Could you check a few things on this model? Use its own coordinates, in mm. Give positions to 0.01 mm unless a question says otherwise; leave off trailing zeros. Loops run counter-clockwise (first coordinate to the right, second up) from the corner with the lowest first, then second, coordinate; pieces in that order, holes last. Notation, with made-up numbers: M 33,13.25 L 49,13.25 A19 cw 49,18.25 Z; hole C -28,58.25 d4. An arc over 180 degrees is marked long. Use a Markdown table: item, result. Add a question column.
1) Suppose I cut it at D-D on y = -2. List the corners of the cut face in (x, z) for me, and give its area (3 significant figures).
2) If I drill on line 1 along Y through (x, z) = (6, 0); line 2 along Z through (x, y) = (3, 0), over which ranges is the centre line in solid material (lowest first)? Write a range as [from, to].
3) Suppose I cut it at C-C on x = 14. List the corners of the cut face in (y, z) for me.
4) Will these pins go through, and if not, where does the flat tip stop? pin 1 Ø2 at (x, y) = (13, -0.5) entering from +Z; pin 2 Ø2 at (x, y) = (4.5, -3) entering from +Z; pin 3 Ø2 at (x, z) = (10.5, 0.5) entering from +Y; pin 4 Ø0.6 at (x, z) = (10, 0) entering from -Y.
5) Suppose I cut it at B-B on z = 1.75. List the corners of the cut face in (x, y) for me, and give its area (3 significant figures).
6) Suppose I cut it at A-A on y = 0. List the corners of the cut face in (x, z) for me.
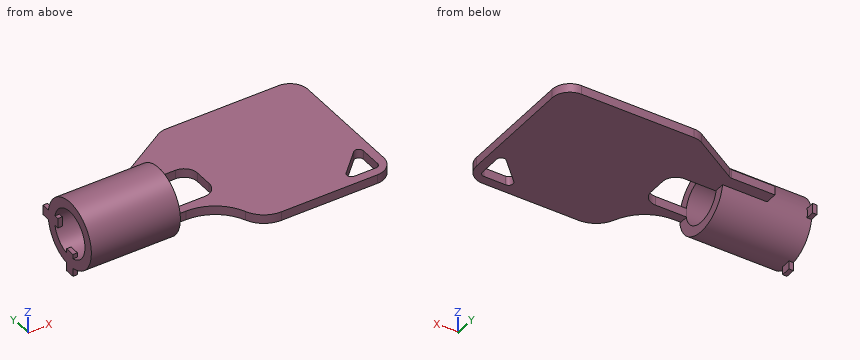
Autodesk Inventor part; units mm, degrees
ref_plane "k_to_1_XY" through (0, 0, 0) normal (1, 0, 0) x (0, 0, -1)
ref_plane "k_to_1_YZ" through (0, 0, 0) normal (0, 0, -1) x (0, 1, 0)
ref_plane "k_to_1_ZX" through (0, 0, 0) normal (0, 1, 0) x (1, 0, 0)
sketch "Sketch_1" plane through (0, 0, 0) normal (1, 0, 0) x (0, 1, 0)
  circle A0 centre (0, 0) radius 3.707
  circle A1 centre (0, 0) radius 2.607
extrude "Extrusion1" add sketch "Sketch_1" along normal blind 10
sketch "Sketch_2" plane through (0, 0, 0) normal (1, 0, 0) x (0, 1, 0)
  line L0 (2.0509, 0.55) -> (2.0509, -0.55)
  line L1 (2.0509, -0.55) -> (4.6009, -0.55)
  line L2 (4.6009, -0.55) -> (4.6009, 0.55)
  line L3 (4.6009, 0.55) -> (2.0509, 0.55)
extrude "Extrusion2" add sketch "Sketch_2" along normal blind 0.5
sketch "Sketch_3" plane through (0, 0, 0) normal (1, 0, 0) x (0, 1, 0)
  line L0 (0.55, -2.0509) -> (-0.55, -2.0509)
  line L1 (-0.55, -2.0509) -> (-0.55, -4.6009)
  line L2 (-0.55, -4.6009) -> (0.55, -4.6009)
  line L3 (0.55, -4.6009) -> (0.55, -2.0509)
extrude "Extrusion3" add sketch "Sketch_3" along normal blind 0.5
sketch "Sketch_4" plane through (0, 0, 0) normal (0, 0, 1) x (1, 0, 0)
  line L0 (5, 5) -> (5, 3.5)
  line L1 (5, 3.5) -> (10, 3.5)
  line L2 (10, 3.5) -> (10, 2.5)
  line L3 (10, 2.5) -> (13.5, 2.5)
  arc A0 (15, 1) -> (13.5, 2.5) centre (13.5, 1) ccw
  line L4 (15, 1) -> (15, -1)
  arc A1 (13.5, -2.5) -> (15, -1) centre (13.5, -1) ccw
  line L5 (13.5, -2.5) -> (10, -2.5)
  line L6 (10, -2.5) -> (10, -3.5)
  line L7 (10, -3.5) -> (10.7881, -3.5)
  arc A2 (15.4232, -6.625) -> (10.7881, -3.5) centre (10.7881, -8.5) ccw
  arc A3 (15.4232, -6.625) -> (18.2043, -8.5) centre (18.2043, -5.5) ccw
  line L8 (18.2043, -8.5) -> (29, -8.5)
  arc A4 (29, -8.5) -> (31, -6.5) centre (29, -6.5) ccw
  line L9 (31, -6.5) -> (31, 6.5)
  arc A5 (31, 6.5) -> (29, 8.5) centre (29, 6.5) ccw
  line L10 (29, 8.5) -> (16.3458, 8.5)
  arc A6 (16.3458, 8.5) -> (15.3109, 8.2114) centre (16.3458, 6.5) ccw
  line L11 (15.3109, 8.2114) -> (10.1193, 5.0721)
  arc A7 (9.8606, 5) -> (10.1193, 5.0721) centre (9.8606, 5.5) ccw
  line L12 (9.8606, 5) -> (5, 5)
  arc A8 (26.7036, -6.6464) -> (27.0571, -7.5) centre (27.0571, -7) ccw
  line L13 (27.0571, -7.5) -> (29.5, -7.5)
  arc A9 (29.5, -7.5) -> (30, -7) centre (29.5, -7) ccw
  line L14 (30, -7) -> (30, -4.5571)
  arc A10 (30, -4.5571) -> (29.1464, -4.2036) centre (29.5, -4.5571) ccw
  line L15 (29.1464, -4.2036) -> (26.7036, -6.6464)
extrude "Extrusion4" add sketch "Sketch_4" along normal mid plane 1
ref_plane "k_to_1_XY" through (0, 0, 0) normal (1, 0, 0) x (0, 0, -1)
ref_plane "k_to_1_YZ" through (0, 0, 0) normal (0, 0, -1) x (0, 1, 0)
ref_plane "k_to_1_ZX" through (0, 0, 0) normal (0, 1, 0) x (1, 0, 0)
ref_plane "3_TO_K_XY" through (27, -6.5, 0) normal (0, 0, 1) x (1, 0, 0)
ref_plane "3_TO_K_YZ" through (27, -6.5, 0) normal (1, 0, 0) x (0, 1, 0)
ref_plane "3_TO_K_ZX" through (27, -6.5, 0) normal (0, 1, 0) x (0, 0, 1)
ref_plane "K1_TO_3_XY" through (29, -3, 0) normal (1, 0, 0) x (0, 0, -1)
ref_plane "K1_TO_3_YZ" through (29, -3, 0) normal (0, 0, -1) x (0, 1, 0)
ref_plane "K1_TO_3_ZX" through (29, -3, 0) normal (0, 1, 0) x (1, 0, 0)
properties part number "LOCNL2_k"
Answer block:
| question | item | result |
|---|---|---|
| 1 | outline | M 0,-3.12 L 10,-3.12 L 10,-1.67 L 0,-1.67 Z; M 0,1.67 L 10,1.67 L 10,3.12 L 0,3.12 Z; M 14.62,-0.5 L 31,-0.5 L 31,0.5 L 14.62,0.5 Z |
| 1 | area | 45.4 mm^2 |
| 2 | line 1 | y = [-3.71, -2.61], [2.61, 5] |
| 2 | line 2 | z = [-3.71, -2.61], [2.61, 3.71] |
| 3 | outline | M -4.67,-0.5 L -2.41,-0.5 L -2.41,0.5 L -4.67,0.5 Z; M 2.41,-0.5 L 7.42,-0.5 L 7.42,0.5 L 2.41,0.5 Z |
| 4 | pin 1 | passes through |
| 4 | pin 2 | stops at z = 3.12 |
| 4 | pin 3 | stops at y = 5.91 |
| 4 | pin 4 | stops at y = -3.71 |
| 5 | outline | M 0,-3.27 L 10,-3.27 L 10,-1.93 L 0,-1.93 Z; M 0,1.93 L 10,1.93 L 10,3.27 L 0,3.27 Z |
| 5 | area | 26.7 mm^2 |
| 6 | outline | M 0,-4.6 L 0.5,-4.6 L 0.5,-3.71 L 10,-3.71 L 10,-2.61 L 0.5,-2.61 L 0.5,-2.05 L 0,-2.05 Z; M 0,2.61 L 10,2.61 L 10,3.71 L 0,3.71 Z; M 15,-0.5 L 31,-0.5 L 31,0.5 L 15,0.5 Z |
